Autodesk Inventor part; units mm, degrees
ref_plane "XZ Plane" through (0, 0, 0) normal (0, 1, 0) x (-1, 0, 0)
ref_plane "XY Plane" through (0, 0, 0) normal (0, 0, 1) x (1, 0, 0)
sketch "Sketch1" plane through (0, 0, 0) normal (0, 0, 1) x (1, 0, 0)
  circle A0 centre (0, 0) radius 65
  dimension "d0" = 130
extrude "Extrusion1" add sketch "Sketch1" along normal blind 25
ref_plane "Work Plane1" through (0, 0, 0) normal (0, 1, 0) x (0, 0, 1)
sketch "Sketch2" plane through (0, 0, 0) normal (0, 1, 0) x (0, 0, 1)
  circle A0 centre (100, 0) radius 100
  line L0 (0, 65) -> (0, -65)
  point P0 (0, 0)
  dimension "d4" = 200
extrude "Extrusion2" cut sketch "Sketch2" along normal mid plane 130
sketch "Sketch3" plane through (0, 0, 0) normal (0, 0, -1) x (-1, 0, 0)
  circle A0 centre (0, 0) radius 65
extrude "Extrusion3" add sketch "Sketch3" along normal blind 10
ref_plane "Work Plane2" through (0, 0, 0) normal (-1, 0, 0) x (0, 0, 1)
properties part number "DiscoSuporteInterno" material "Nickel-Copper Alloy 400"
Design review of the part built by this model. Coordinates are the model's own, in mm. Round coordinates to 2 decimals unless told otherwise and drop trailing zeros. Write each loop counter-clockwise with the first axis right and the second up, starting at its lowest first coordinate (ties: lowest second). Pieces come first, ordered by that corner, then holes.
Item 1: The part is to be moulded in two halves that separate along X. For faces 1 (the flat face through (1, 1, -10)), 2 (the cylindrical face through (-0.987, -0.916, 0.005)), 3 (the cylindrical face through (-57.31, 30.67, 3.46)), say which applies: +X half, -X half, draft (parallel to the pull), parting line (faces both ways), or undercut.
Item 2: We need section C-C on x = 39. Write out the cut boundary in (y, z), and give its area (3 significant figures).
Item 3: We need section D-D on z = 22.5. Write out the cut boundary in (x, y).
Item 4: We need section B-B on y = -3. Write out the cut boundary in (x, z).
Item 5: We need section A-A on z = 13. Write out the cut boundary in (x, y), and give its area (3 significant figures).
Item 6: For probe 1 along X at (y, z) = (41, 11); probe 2 along X at (y, z) = (4.5, 21.5); probe 3 along Z at (x, y) = (2.5, 14), list the stretches that pass through material, from the lowest coordinate up.
Item 7: Clearance check with flat-ended pins moving along their axes: pin 1 Ø10 at (x, y) = (-51, 24.5) entering from +Z; pin 2 Ø2 at (y, z) = (17, 14.5) entering from -X; pin 3 Ø4 at (y, z) = (35, 9) entering from -X. State where each tip first meets the part, or that it passes through.
Returned:
1. face 1: draft
1. face 2: undercut
1. face 3: parting line
2. outline: (-52, -10) - (52, -10) - (52, 7.92) - (-52, 7.92) - close
2. area: 1,860 mm2
3. outline: (-63.2, -15.21) - (-63.2, 15.21) arc R65 ccw to start; (63.2, -15.21) arc R65 ccw to (63.2, 15.21) - close
4. outline: (-64.93, -10) - (64.93, -10) - (64.93, 23.95) arc R100 cw to (-64.93, 23.95) - close
5. outline: (-49.31, -42.36) - (-49.31, 42.36) arc R65 ccw to start; (49.31, -42.36) arc R65 ccw to (49.31, 42.36) - close
5. area: 1,820 mm2
6. probe 1: x = -50.44 to -45.6, 45.6 to 50.44
6. probe 2: x = -64.84 to -61.95, 61.95 to 64.84
6. probe 3: z = -10 to 0.03
7. pin 1: stops at z = 17.15
7. pin 2: stops at x = -63
7. pin 3: stops at x = -56
